Verification items for the finished model (mm, model axes). A direction names the side the tool comes from. Round coordinates to 2 decimals unless told otherwise and drop trailing zeros. Write each loop counter-clockwise with the first axis right and the second up, starting at its lowest first coordinate (ties: lowest second). Pieces come first, ordered by that corner, then holes. Notation, with made-up numbers: M 31,20 L 40,20 A29 ccw 40,53 Z; hole C -40,58 d3. An arc over 180 degrees is marked long. Answer in a Markdown table with one row per item. Add a question column.
1. Sectioned sample at B-B on z = -5. Record the cut outline in (x, y).
2. Set-up check for faces 1 (the flat face through (0, -153, -13.5)), 2 (the flat face through (15, -153, 0)): record each of +Z, -Z, +X, -X, +Y, -Y from which the full face is reachable in a straight line by a thin tool's end or side.
3. Sectioned sample at A-A on x = 3. Record the cut outline in (y, z).
4. Draft check along Z on faces 3 (the flat face through (0, -153, 15)), 4 (the flat face through (0, -153, 13.5)), 5 (the cylindrical face through (-14, -153, -13)). Enter one of: pulls with the +Z half, pulls with the -Z half, needs draft (parallel to the pull), parting line crosses it, or undercut.
5. Go/stop test with a flat-tipped pin: pin 1 Ø12 at (x, z) = (-11, 0) entering from -Y. Record where the tip stops, or that it passes through.
6. Sectioned sample at C-C on y = -272. Record the cut outline in (x, z).
7. Material ranges on probe 1 along X at (y, z) = (-90.5, 8); probe 2 along Z at (x, y) = (5, -23), recorded low to high.
```python
from build123d import *

# Parameters (mm, degrees)
F1_DEPTH = 310
F3_DEPTH = 30.001


with BuildPart() as f1:
    # F0 (on Front) → F1 (new body)
    with BuildSketch(Plane.XZ):
        with BuildLine():
            Line((-10, -15), (10, -15))
            ThreePointArc((10, -15), (13.535534, -13.535534), (15, -10))
            Line((15, -10), (15, 10))
            ThreePointArc((15, 10), (13.535534, 13.535534), (10, 15))
            Line((10, 15), (-10, 15))
            ThreePointArc((-10, 15), (-13.535534, 13.535534), (-15, 10))
            Line((-15, 10), (-15, -10))
            ThreePointArc((-15, -10), (-13.535534, -13.535534), (-10, -15))
        make_face()
        with BuildLine():
            ThreePointArc((-10, -13.5), (-12.474874, -12.474874), (-13.5, -10))
            Line((-13.5, -10), (-13.5, 10))
            ThreePointArc((-13.5, 10), (-12.474874, 12.474874), (-10, 13.5))
            Line((-10, 13.5), (10, 13.5))
            ThreePointArc((10, 13.5), (12.474874, 12.474874), (13.5, 10))
            Line((13.5, 10), (13.5, -10))
            ThreePointArc((13.5, -10), (12.474874, -12.474874), (10, -13.5))
            Line((10, -13.5), (-10, -13.5))
        make_face(mode=Mode.SUBTRACT)
    extrude(amount=F1_DEPTH)

    # F2 (on face) → F3 (cut, through all)
    with BuildSketch(Plane.YZ.offset(15)):
        Polygon((0, -15), (0, 15), (-30, -15), align=None)
        Polygon((-310, 15), (-310, -15), (-280, -15), align=None)
    extrude(amount=-F3_DEPTH, mode=Mode.SUBTRACT)


solid = f1.part
```
Geometry check:
| question | item | result |
|---|---|---|
| 1 | outline | M -15,-290 L -13.5,-290 L -13.5,-20 L -15,-20 Z; M 13.5,-290 L 15,-290 L 15,-20 L 13.5,-20 Z |
| 2 | face 1 | +Y, -Y |
| 2 | face 2 | +Z, -Z, +X, +Y, -Y |
| 3 | outline | M -310,15 L -308.5,13.5 L -1.5,13.5 L 0,15 Z; M -281.5,-13.5 L -280,-15 L -30,-15 L -28.5,-13.5 Z |
| 4 | face 3 | pulls with the +Z half |
| 4 | face 4 | undercut |
| 4 | face 5 | pulls with the -Z half |
| 5 | pin 1 | stops at y = -300.45 |
| 6 | outline | M -15,-10 A5 ccw -10,-15 L 10,-15 A5 ccw 15,-10 L 15,10 A5 ccw 10,15 L -10,15 A5 ccw -15,10 Z; hole M -13.5,-10 A3.5 ccw -10,-13.5 L 10,-13.5 A3.5 ccw 13.5,-10 L 13.5,10 A3.5 ccw 10,13.5 L -10,13.5 A3.5 ccw -13.5,10 Z |
| 7 | probe 1 | x = -15 to -13.5, 13.5 to 15 |
| 7 | probe 2 | z = 13.5 to 15 |
